Input: part model. Units: mm. Frame: model coordinates. Face numbers are marked on the shaded views. A direction names the side the tool comes from. Round coordinates to 2 decimals unless told otherwise and drop trailing zeros. Loops run counter-clockwise (first coordinate to the right, second up) from the corner with the lowest first, then second, coordinate; pieces in that order, holes last. Notation, with made-up numbers: (-28, 15.25) -> (30, 15.25) arc R13 ccw to (30, 40.25) -> close; hole circle Ø2 at (62, 44). An arc over 180 degrees is marked (long way). Answer as a JSON object with one key per item and string values. Group by question number.
Item 1: Set-up query: the marked faces 1 and 2. Return all of +Z, -Z, +X, -X, +Y, -Y with unobstructed straight access to the full face (end or side cutting, diameter ignored); none if empty.
Item 2: Material intervals for line 1 (Y direction, x = 22, z = 23.75); line 2 (X direction, y = 12.15, z = 10.5); line 3 (Z direction, x = 15.25, y = -9), sorted ascending. Write a range as [from, to].
Item 3: Draft query along Y for the marked faces 3, 4 and 5. Return one class per face: released by +Y, released by -Y, zero draft, split by the parting line, or undercut.
Item 4: Section query A-A on z = 18.5. Return loops of the section in (x, y), and give its area (3 significant figures).
Item 5: Pin query (flat end, axial travel): pin 1 (4 mm diameter, centred on x = 19.5, y = 8, fed in from +Z); pin 2 (2 mm diameter, centred on x = 17, y = 2.5, fed in from +Z); pin 3 (0.7 mm diameter, centred on x = 19.5, z = 10.5, fed in from -Y) (3 decimals). Return the tip coordinate at first contact, or that it passes through.
Item 6: Section query D-D on x = 21. Return loops of the section in (y, z).
Item 7: Section query B-B on x = 19.5. Return loops of the section in (y, z).
Item 8: Section query C-C on z = 10.5. Return loops of the section in (x, y).
from build123d import *

# Parameters (mm, degrees)
SKETCH023_W     = 10.9
SKETCH023_H     = 29
PAD007_DEPTH    = 2.8
SKETCH024_W     = 10.9
SKETCH024_H     = 2.8
PAD008_DEPTH    = 15.6
CHAMFER_SIZE    = 2.8
SKETCH025_R     = 0.6
POCKET014_DEPTH = 29.001


with BuildPart() as part:
    # Sketch023 (on DatumPlane) → Pad007 (new body)
    with BuildSketch(Plane.XY.offset(7)):
        with Locations((19.95, 0)):
            Rectangle(SKETCH023_W, SKETCH023_H)
    extrude(amount=PAD007_DEPTH)

    # Sketch024 (on DatumPlane) → Pad008 (join)
    with BuildSketch(Plane.XY.offset(9.8)):
        with Locations((19.95, -13.1)):
            Rectangle(SKETCH024_W, SKETCH024_H)
        with Locations((19.95, 13.1)):
            Rectangle(SKETCH024_W, SKETCH024_H)
    extrude(amount=PAD008_DEPTH)

    # Chamfer
    chamfer_edges = [part.edges().sort_by_distance(p)[0] for p in [
        (19.95, 11.7, 9.8),
        (19.95, -11.7, 9.8),
    ]]
    chamfer(chamfer_edges, length=CHAMFER_SIZE)

    # Sketch025 (on DatumPlane) → Pocket014 (cut, through all)
    with BuildSketch(Plane.XZ.offset(14.5)):
        with Locations((19.5, 10.5)):
            Circle(SKETCH025_R)
    extrude(amount=-POCKET014_DEPTH, mode=Mode.SUBTRACT)


solid = part.part
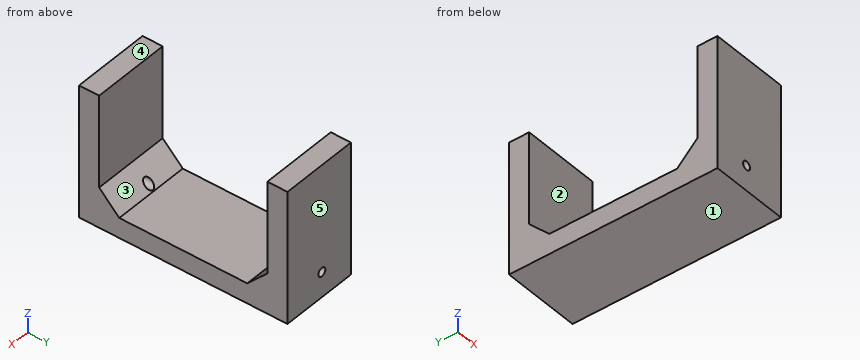
Solved:
{
 "1": {"face 1": "-Z, +X, -X, +Y, -Y", "face 2": "+Z, +X, -X"},
 "2": {"line 1": "[-14.5, -11.7], [11.7, 14.5]", "line 2": "[14.5, 18.9], [20.1, 25.4]", "line 3": "[7, 9.9]"},
 "3": {"face 3": "undercut", "face 4": "zero draft", "face 5": "released by +Y"},
 "4": {"outline": "(14.5, -14.5) -> (25.4, -14.5) -> (25.4, -11.7) -> (14.5, -11.7) -> close; (14.5, 11.7) -> (25.4, 11.7) -> (25.4, 14.5) -> (14.5, 14.5) -> close", "area": "61.0 mm²"},
 "5": {"pin 1": "z = 10.84", "pin 2": "z = 9.8", "pin 3": "through"},
 "6": {"outline": "(-14.5, 7) -> (14.5, 7) -> (14.5, 25.4) -> (11.7, 25.4) -> (11.7, 12.6) -> (8.9, 9.8) -> (-8.9, 9.8) -> (-11.7, 12.6) -> (-11.7, 25.4) -> (-14.5, 25.4) -> close"},
 "7": {"outline": "(-14.5, 7) -> (14.5, 7) -> (14.5, 9.9) -> (9, 9.9) -> (8.9, 9.8) -> (-8.9, 9.8) -> (-9, 9.9) -> (-14.5, 9.9) -> close; (-14.5, 11.1) -> (-10.2, 11.1) -> (-11.7, 12.6) -> (-11.7, 25.4) -> (-14.5, 25.4) -> close; (10.2, 11.1) -> (14.5, 11.1) -> (14.5, 25.4) -> (11.7, 25.4) -> (11.7, 12.6) -> close"},
 "8": {"outline": "(14.5, -14.5) -> (18.9, -14.5) -> (18.9, -9.6) -> (14.5, -9.6) -> close; (14.5, 9.6) -> (18.9, 9.6) -> (18.9, 14.5) -> (14.5, 14.5) -> close; (20.1, -14.5) -> (25.4, -14.5) -> (25.4, -9.6) -> (20.1, -9.6) -> close; (20.1, 9.6) -> (25.4, 9.6) -> (25.4, 14.5) -> (20.1, 14.5) -> close"}
}
